Autodesk Inventor part; units mm, degrees
ref_plane "YZ Plane" through (0, 0, 0) normal (1, 0, 0) x (0, 1, 0)
ref_plane "XZ Plane" through (0, 0, 0) normal (0, 1, 0) x (-1, 0, 0)
ref_plane "XY Plane" through (0, 0, 0) normal (0, 0, 1) x (1, 0, 0)
sketch "Sketch1" plane through (0, 0, 0) normal (0, 0, 1) x (1, 0, 0)
  line L0 (0, 0) -> (25.4, 0)
  line L1 (25.4, 0) -> (25.4, 76.2)
  line L2 (25.4, 76.2) -> (0, 76.2)
  line L3 (0, 76.2) -> (0, 0)
  line L4 (25.4, 76.2) -> (50.8, 76.2)
  line L5 (50.8, 76.2) -> (50.8, 50.8)
  line L6 (50.8, 50.8) -> (25.4, 50.8)
  line L7 (25.4, 50.8) -> (25.4, 76.2)
  line L8 (0, 76.2) -> (-25.4, 76.2)
  line L9 (-25.4, 76.2) -> (-25.4, 50.8)
  line L10 (-25.4, 50.8) -> (0, 50.8)
  line L11 (0, 50.8) -> (0, 76.2)
  dimension "d0" = 25.4
  dimension "d1" = 76.2
  dimension "d2" = 25.4
  dimension "d3" = 25.4
  dimension "d4" = 25.4
  dimension "d5" = 25.4
extrude "Extrusion1" add sketch "Sketch1" along normal blind 3.175
sketch "Sketch2" plane through (0, 0, 3.175) normal (0, 0, 1) x (1, 0, 0)
  line L0 (-25.4, 76.2) -> (-25.4, 50.8) construction
  line L1 (-25.4, 63.5) -> (-12.7, 63.5) construction
  line L2 (-12.7, 63.5) -> (12.7, 63.5) construction
  line L3 (12.7, 63.5) -> (38.1, 63.5) construction
  line L4 (12.7, 63.5) -> (12.7, 38.1) construction
  line L5 (12.7, 38.1) -> (12.7, 12.7) construction
  circle A0 centre (-12.7, 63.5) radius 2.5797
  circle A1 centre (12.7, 63.5) radius 2.5797
  circle A2 centre (38.1, 63.5) radius 2.5797
  circle A3 centre (12.7, 38.1) radius 2.5797
  circle A4 centre (12.7, 12.7) radius 2.5797
  point P0 (0, 0)
  dimension "d8" = 12.7
  dimension "d9" = 25.4
  dimension "d10" = 25.4
  dimension "d11" = 25.4
  dimension "d12" = 25.4
  dimension "d13" = 5.1594
extrude "Extrusion2" cut sketch "Sketch2" against normal blind 3.175
fillet "Fillet1" radius 3.175 8 edges at (50.8, 76.2, 1.5875) (50.8, 50.8, 1.5875) (25.4, 50.8, 1.5875) (25.4, 0, 1.5875) (0, 0, 1.5875) (0, 50.8, 1.5875) (-25.4, 50.8, 1.5875) (-25.4, 76.2, 1.5875)
properties part number "0.125 T-Gusset"
Could you check a few things on this model? Use its own coordinates, in mm. A direction names the side the tool comes from. Round coordinates to 2 decimals unless told otherwise and drop trailing zeros. Write each loop counter-clockwise with the first axis right and the second up, starting at its lowest first coordinate (ties: lowest second). Pieces come first, ordered by that corner, then holes.
(1) For pin 1 (12 mm diameter, centred on x = 37, y = 32, fed in from +Z); pin 2 (1.6 mm diameter, centred on y = 27.5, z = 1.5, fed in from +X), each with a flat end and sliding along its axis, tell me the tip position at first contact or that it passes through.
Findings below:
pin 1: passes through
pin 2: stops at x = 25.4
(2) Suppose I cut it at B-B on z = 2.65. Write out the boundary of the cut face in (x, y) (3 decimals).
Findings below:
outline: (-25.4, 53.975) arc R3.175 ccw to (-22.225, 50.8) - (-3.175, 50.8) arc R3.175 cw to (0, 47.625) - (0, 3.175) arc R3.175 ccw to (3.175, 0) - (22.225, 0) arc R3.175 ccw to (25.4, 3.175) - (25.4, 47.625) arc R3.175 cw to (28.575, 50.8) - (47.625, 50.8) arc R3.175 ccw to (50.8, 53.975) - (50.8, 73.025) arc R3.175 ccw to (47.625, 76.2) - (-22.225, 76.2) arc R3.175 ccw to (-25.4, 73.025) - close; hole circle Ø5.159 at (-12.7, 63.5); hole circle Ø5.159 at (12.7, 12.7); hole circle Ø5.159 at (12.7, 38.1); hole circle Ø5.159 at (12.7, 63.5); hole circle Ø5.159 at (38.1, 63.5)
(3) Suppose I cut it at C-C on y = 12.7. Write out the boundary of the cut face in (x, z) (3 decimals).
Findings below:
outline: (0, 0) - (10.12, 0) - (10.12, 3.175) - (0, 3.175) - close; (15.28, 0) - (25.4, 0) - (25.4, 3.175) - (15.28, 3.175) - close
(4) Which directions (+Z, -Z, +X, -X, +Y, -Y) give clear straight access to the entire face, cutting with the end or side of a thin tool? Please do faces 4 (the face through (-24.45, 75.29, 1.61)), 5 (the face through (38, 50.8, 2)).
Findings below:
face 4: +Z, -Z, -X, +Y
face 5: +Z, -Z, +X, -Y
(5) Thinking about a two-plate mould opening in X: for faces 1 (the face through (49.85, 51.71, 1.61)), 2 (the face through (-11.313, 65.675, 1.61)), 3 (the face through (13, 0, 2)), which applies, +X half, -X half, draft (parallel to the pull), parting line (faces both ways), or undercut?
Findings below:
face 1: +X half
face 2: undercut
face 3: draft
(6) Suppose I cut it at A-A on x = 12.7. Write out the boundary of the cut face in (y, z) (3 decimals), and give its area (3 significant figures).
Findings below:
outline: (0, 0) - (10.12, 0) - (10.12, 3.175) - (0, 3.175) - close; (15.28, 0) - (35.52, 0) - (35.52, 3.175) - (15.28, 3.175) - close; (40.68, 0) - (60.92, 0) - (60.92, 3.175) - (40.68, 3.175) - close; (66.08, 0) - (76.2, 0) - (76.2, 3.175) - (66.08, 3.175) - close
area: 193 mm2
(7) Suppose I cut it at D-D on x = -12.7. Write out the boundary of the cut face in (y, z) (3 decimals).
Findings below:
outline: (50.8, 0) - (60.92, 0) - (60.92, 3.175) - (50.8, 3.175) - close; (66.08, 0) - (76.2, 0) - (76.2, 3.175) - (66.08, 3.175) - close
(8) If I drill on probe 1 along Y at (x, z) = (12.7, 2.2); probe 2 along Y at (x, z) = (38.1, 1.9); probe 3 along Y at (x, z) = (41.5, 2.2), over which ranges is the centre line in solid material (lowest first)?
Findings below:
probe 1: y = 0 to 10.12, 15.28 to 35.52, 40.68 to 60.92, 66.08 to 76.2
probe 2: y = 50.8 to 60.92, 66.08 to 76.2
probe 3: y = 50.8 to 76.2
